Input: part model. Units: mm. Frame: model coordinates. Face numbers are marked on the shaded views. A direction names the side the tool comes from. Coordinates: 2 decimals unless noted, no trailing zeros. Order: outer loops, then holes, each group sorted by start corner. A loop starts at its lowest first (then second) coordinate and runs counter-clockwise, first axis right, second up.
Autodesk Inventor part; units mm, degrees
ref_plane "YZ Plane" through (0, 0, 0) normal (1, 0, 0) x (0, 1, 0)
ref_plane "XZ Plane" through (0, 0, 0) normal (0, 1, 0) x (-1, 0, 0)
ref_plane "XY Plane" through (0, 0, 0) normal (0, 0, 1) x (1, 0, 0)
sketch "Sketch1" plane through (0, 0, 0) normal (0, 0, 1) x (1, 0, 0)
  line L0 (9.6801, -14.008) -> (7.2052, -11.5331) construction
  line L1 (7.2052, -11.5331) -> (11.5893, -7.1491) construction
  line L2 (11.5893, -7.1491) -> (14.0642, -9.6239) construction
  line L3 (14.0642, -9.6239) -> (9.6801, -14.008) construction
  arc A0 (12.6369, -4.7496) -> (4.7496, -12.6369) centre (0, 0) ccw construction
  line L4 (10.9298, -3.0424) -> (12.6369, -4.7496) construction
  line L5 (11.6618, -4.6122) -> (10.9298, -3.0424) construction
  arc A1 (11.6618, -4.6122) -> (10.8551, -4.47) centre (11.2086, -4.8235) ccw construction
  line L6 (10.7915, -4.5335) -> (10.8551, -4.47) construction
  arc A2 (10.7915, -4.5335) -> (10.6527, -4.9738) centre (11.1451, -4.887) ccw construction
  line L7 (10.915, -6.4612) -> (10.6527, -4.9738) construction
  arc A3 (10.7761, -6.9016) -> (10.915, -6.4612) centre (10.4226, -6.548) ccw construction
  line L8 (6.9016, -10.7761) -> (10.7761, -6.9016) construction
  arc A4 (6.4612, -10.915) -> (6.9016, -10.7761) centre (6.548, -10.4226) ccw construction
  line L9 (6.4612, -10.915) -> (4.9738, -10.6527) construction
  arc A5 (4.9738, -10.6527) -> (4.5335, -10.7915) centre (4.887, -11.1451) ccw construction
  line L10 (4.5335, -10.7915) -> (4.47, -10.8551) construction
  arc A6 (4.47, -10.8551) -> (4.6122, -11.6618) centre (4.8235, -11.2086) ccw construction
  line L11 (4.6122, -11.6618) -> (3.0424, -10.9298) construction
  line L12 (3.0424, -10.9298) -> (4.7496, -12.6369) construction
  line L13 (-1.7167, -14.6498) -> (-1.7167, -17.5) construction
  line L14 (-1.7167, -17.5) -> (1.7167, -17.5) construction
  line L15 (1.7167, -14.6498) -> (1.7167, -17.5) construction
  arc A7 (1.7167, -14.6498) -> (6.9595, -13.0049) centre (0, 0) ccw construction
  arc A8 (6.9595, -13.0049) -> (8.2728, -15.1789) centre (8.2994, -13.6792) ccw construction
  line L16 (8.2728, -15.1789) -> (7.6816, -15.1684) construction
  arc A9 (8.5249, -17.8901) -> (7.6816, -15.1684) centre (7.655, -16.6682) ccw construction
  line L17 (8.5249, -17.8901) -> (13.5161, -14.3366) construction
  line L18 (13.5161, -14.3366) -> (13.5161, -12.2823) construction
  line L19 (13.5161, -12.2823) -> (14.6168, -12.2823) construction
  line L20 (14.6168, -12.2823) -> (14.6168, -1.9776) construction
  arc A10 (14.6168, -1.9776) -> (1.7167, 14.6498) centre (0, 0) ccw construction
  line L21 (1.7167, 14.6498) -> (1.7167, 17.5) construction
  line L22 (-1.7167, 17.5) -> (1.7167, 17.5) construction
  line L23 (-1.7167, 14.6498) -> (-1.7167, 17.5) construction
  arc A11 (-1.7167, 14.6498) -> (-14.2817, -3.6872) centre (0, 0) ccw construction
  line L24 (-14.2817, -3.6872) -> (-15.4135, -5.7935) construction
  arc A12 (-15.4135, -5.7935) -> (-14.5984, -8.502) centre (-13.6517, -6.7402) ccw construction
  line L25 (-14.5984, -8.502) -> (-9.6326, -11.1703) construction
  arc A13 (-9.6326, -11.1703) -> (-1.7167, -14.6498) centre (0, 0) ccw construction
  line L26 (-24.6, 24.6) -> (25.2, -25.2) construction
  line L27 (25.2, 24.6) -> (-24.6, -25.2) construction
  arc A14 (-1.4283, 10.15) -> (-9.5043, -3.8381) centre (0, 0) ccw
  circle A15 centre (0, 0) radius 10.1 construction
  line L28 (-1.4283, 10.15) -> (1.4283, 10.15)
  line L29 (-8.076, -6.3119) -> (-9.5043, -3.8381)
  line L30 (9.5043, -3.8381) -> (8.076, -6.3119)
  arc A16 (1.4283, 10.15) -> (-1.4283, 10.15) centre (0, 0) ccw
  arc A17 (9.5043, -3.8381) -> (1.4283, 10.15) centre (0, 0) ccw
  arc A18 (8.076, -6.3119) -> (9.5043, -3.8381) centre (0, 0) ccw
  arc A19 (-8.076, -6.3119) -> (8.076, -6.3119) centre (0, 0) ccw
  arc A20 (-9.5043, -3.8381) -> (-8.076, -6.3119) centre (0, 0) ccw
  arc A21 (10.7054, -6.8309) -> (10.8165, -6.4786) centre (10.4226, -6.548) ccw
  line L31 (10.8165, -6.4786) -> (10.5542, -4.9912)
  arc A22 (10.7208, -4.4628) -> (10.5956, -4.6461) centre (11.1451, -4.887) ccw construction
  line L32 (10.7208, -4.4628) -> (10.7844, -4.3992) construction
  arc A23 (11.7601, -5.0598) -> (10.7844, -4.3992) centre (11.2086, -4.8235) ccw construction
  line L33 (11.7601, -5.0598) -> (10.5994, -2.5707) construction
  line L34 (10.5994, -2.5707) -> (12.5972, -4.5684) construction
  arc A24 (12.5972, -4.5684) -> (4.5684, -12.5972) centre (0, 0) ccw construction
  line L35 (4.5684, -12.5972) -> (2.5707, -10.5994) construction
  line L36 (2.5707, -10.5994) -> (4.2491, -11.3821) construction
  arc A25 (4.3992, -10.7844) -> (4.2491, -11.3821) centre (4.8235, -11.2086) ccw construction
  line L37 (4.3992, -10.7844) -> (4.4628, -10.7208) construction
  arc A26 (4.9912, -10.5542) -> (4.6461, -10.5956) centre (4.887, -11.1451) ccw
  line L38 (4.9912, -10.5542) -> (6.4786, -10.8165)
  arc A27 (6.4786, -10.8165) -> (6.8309, -10.7054) centre (6.548, -10.4226) ccw
  line L39 (6.8309, -10.7054) -> (10.7054, -6.8309)
  circle A28 centre (0, 0) radius 11.5695
  arc A29 (4.6461, -10.5956) -> (4.4628, -10.7208) centre (4.887, -11.1451) ccw construction
  arc A30 (10.5956, -4.6461) -> (10.5542, -4.9912) centre (11.1451, -4.887) ccw
  line L40 (14.8492, -10.3238) -> (10.3238, -14.8492)
  line L41 (14.8492, -10.3238) -> (14.8492, -4.8738)
  line L42 (14.8492, -4.8738) -> (10.5631, 4.7195)
  line L43 (10.3238, -14.8492) -> (4.8738, -14.8492)
  line L44 (4.8738, -14.8492) -> (-4.7195, -10.5631)
  dimension "d4" = 20.2
  dimension "d5" = 10.15
  dimension "d6" = 20.5
  dimension "d9" = 360
  dimension "d11" = 0.1
  dimension "d31" = 6.4
  dimension "d32" = 17.8
  dimension "d33" = 3.2
  dimension "d34" = 135
  dimension "d35" = 5.45
  dimension "d36" = 5.45
extrude "Extrusion1" add sketch "Sketch1" against normal blind 5 contours A16 L28 | L29 A20 | A18 L30 | L39 A27 L38 A26 A28 A30 L31 A21 | A21 L31 A30 A28 L42 L41 L40 L43 L44 A26 L38 A27 L39 | A28
sketch "Sketch3" plane through (0, 0, -5) normal (0, 0, -1) x (-1, 0, 0)
  line L0 (9.5043, -3.8381) -> (8.076, -6.3119)
  arc A0 (-8.076, -6.3119) -> (8.076, -6.3119) centre (0, 0) ccw
  line L1 (-8.076, -6.3119) -> (-9.5043, -3.8381)
  arc A1 (-1.4283, 10.15) -> (-9.5043, -3.8381) centre (0, 0) ccw
  line L2 (-1.4283, 10.15) -> (1.4283, 10.15)
  arc A2 (9.5043, -3.8381) -> (1.4283, 10.15) centre (0, 0) ccw
  arc A3 (4.7195, -10.5631) -> (-10.5631, 4.7195) centre (0, 0) ccw
  circle A4 centre (0, 0) radius 8
  circle A5 centre (0, 0) radius 10.25
  line L3 (-10.5631, 4.7195) -> (-14.8492, -4.8738)
  line L4 (-14.8492, -4.8738) -> (-14.8492, -10.3238)
  line L5 (-14.8492, -10.3238) -> (-10.3238, -14.8492)
  line L6 (-10.3238, -14.8492) -> (-4.8738, -14.8492)
  line L7 (-4.8738, -14.8492) -> (4.7195, -10.5631)
  dimension "d17" = 16
extrude "Extrusion3" add sketch "Sketch3" along normal blind 4 contours A5 L0 | L0 A0 L1 A1 L2 A2 | A5 L1 | L2 A5 | L7 L6 L5 L4 L3 A3
sketch "Sketch4" plane through (10.6492, -14.5238, 0) normal (0.7071, -0.7071, 0) x (0, 0, -1)
  line L0 (0, 0) -> (0, 5.4794) construction
  line L1 (0, 0) -> (9, 0) construction
  line L2 (0, 5.4794) -> (9, 5.4794) construction
  line L3 (0, 2.7397) -> (9, 2.7397) construction
  circle A0 centre (7.2, 2.7397) radius 1.4
  line L4 (9, 5.4794) -> (9, 0)
  dimension "d20" = 2.8
extrude "Extrusion4" cut sketch "Sketch4" against normal up to surface
properties part number "30_focus_inlet_objective_mount_deltastage_v7"
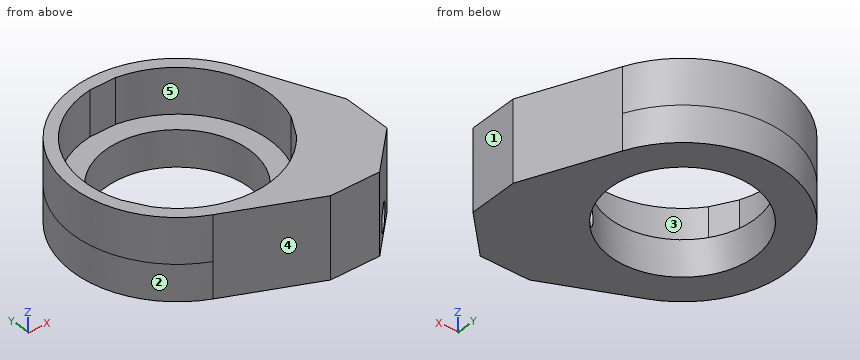
Item 1: Pin query (flat end, axial travel): pin 1 Ø3 at (x, z) = (-2, -4.5) entering from -Y; pin 2 Ø5 at (y, z) = (-3.5, -4) entering from +X; pin 3 Ø3 at (x, z) = (0.5, -3.5) entering from -Y; pin 4 Ø2 at (y, z) = (-6, -3.5) entering from -X. Return the tip coordinate at first contact, or that it passes through.
Response values:
pin 1: stops at y = -12.45
pin 2: stops at x = 14.85
pin 3: stops at y = -13.57
pin 4: stops at x = -10.43
Item 2: Cut plane D-D on x = 0.75. Return loops of the section in (y, z).
Response values:
outline: (-13.01, -9) - (-7.96, -9) - (-7.96, -5) - (-10.22, -5) - (-10.22, 0) - (-13.01, 0) - close; (7.96, -9) - (11.55, -9) - (11.55, 0) - (10.15, 0) - (10.15, -5) - (7.96, -5) - close
Item 3: Access query for the marked faces 4 and 5. Directions: +Z, -Z, +X, -X, +Y, -Y. A direction counts if a zero-diameter tool reaches every point of the face in a straight line with its end or side. Return the directions, or none.
Response values:
face 4: +Z, -Z, -X, -Y
face 5: +Z
Item 4: Draft query along X for the marked faces 1, 2 and 3. Return one class per face: pulls with the +X half, pulls with the -X half, needs draft (parallel to the pull), parting line crosses it, or undercut.
Response values:
face 1: pulls with the +X half
face 2: parting line crosses it
face 3: undercut
Item 5: Cut plane C-C on z = -7.75. Return loops of the section in (x, y), then the cut area to 3 significant figures.
Response values:
outline: (-4.72, -10.56) - (4.87, -14.85) - (10.32, -14.85) - (11.68, -13.5) - (4.67, -6.49) arc R8 cw (long way) to (6.49, -4.67) - (13.5, -11.68) - (14.85, -10.32) - (14.85, -4.87) - (10.56, 4.72) arc R11.57 ccw (long way) to start
area: 292 mm2
Item 6: Cut plane A-A on x = -5.5. Return loops of the section in (y, z), then the cut area to 3 significant figures.
Response values:
outline: (-10.18, -9) - (-5.81, -9) - (-5.81, -5) - (-8.65, -5) - (-8.65, 0) - (-10.18, 0) - close; (5.81, -9) - (10.18, -9) - (10.18, 0) - (8.65, 0) - (8.65, -5) - (5.81, -5) - close
area: 50.2 mm2
Item 7: Ray query, probe 1 along Y at (x, z) = (0, -6.7); probe 2 along X at (y, z) = (9.5, -4.5); probe 3 along X at (y, z) = (2, -3.5). Return the intervals inside material, ascending.
Response values:
probe 1: y = -12.67 to -8, 8 to 11.57
probe 2: x = -6.6 to -3.85, 3.85 to 6.6
probe 3: x = -11.4 to -10.05, 10.05 to 11.78
Item 8: Cut plane B-B on y = 2.5. Return loops of the section in (x, z), then the cut area to 3 significant figures.
Response values:
outline: (-11.3, -9) - (-7.6, -9) - (-7.6, -5) - (-9.94, -5) - (-9.94, 0) - (-11.3, 0) - close; (7.6, -9) - (11.55, -9) - (11.55, 0) - (9.94, 0) - (9.94, -5) - (7.6, -5) - close
area: 45.5 mm2
